For this review, take the finished solid that the model builds, in its own axes (mm). A direction names the side the tool comes from. Round coordinates to 2 decimals unless told otherwise and drop trailing zeros. Write each loop counter-clockwise with the first axis right and the second up, starting at its lowest first coordinate (ties: lowest second). Pieces come first, ordered by that corner, then holes. Notation, with made-up numbers: M 72,-37.75 L 77,-37.75 A21 cw 77,-4.75 Z; hole C 68.5,-32 d2. An arc over 180 degrees is marked long. Use one line per item in the form item = value. Start each with the question number.
Item 1: Add section B-B (x = -88.5). State the section outline as (y, z) points, and give its area (3 significant figures).
Item 2: Add section C-C (y = -21). State the section outline as (x, z) points (1 decimal), and give its area (3 significant figures).
Item 3: For line 1 (Y direction, x = -102, z = -24.5); line 2 (Z direction, x = -55.5, y = -8); line 3 (X direction, y = -12, z = -7.5), list the stretches that pass through material, from the lowest coordinate up. Write a range as [from, to].
Item 4: Add section A-A (z = 3.5). State the section outline as (x, y) points, and give its area (3 significant figures).
Item 5: For P1, Ø3, axis at y = -6.5, z = 33, coming from the -X side; P2, Ø12, axis at y = -48, z = 24, coming from the -X side; P3, Ø2, axis at x = -102, y = -9, coming from the +Z side; P4, Ø4, axis at x = -31, y = -16, coming from the +Z side, all flat-tipped, find the tip position at first contact; note any pin that passes through.
Item 6: For faces 5 (the cylindrical face through (-59.555, -37.744, -48.236)), 6 (the cylindrical face through (-68.197, -6.261, -30.855)), list the 3-axis set-ups (+Z, -Z, +X, -X, +Y, -Y) from which the entire face can be reached by the end or side of a thin tool; tool diameter is ignored.
Item 7: Draft analysis for pull direction X (two halves, no side actions). For faces 1 (the cylindrical face through (-100.82, -37.74, 23.23)), 2 (the cylindrical face through (-18.292, -37.744, 23.233)), 3 (the cylindrical face through (-101.66, -6.26, -30.8)), 4 (the flat face through (-39, 0, 23)), state which applies: released by +X, released by -X, zero draft, split by the parting line, or undercut.
Item 8: Add section D-D (y = -7). State the section outline as (x, z) points, and give its area (3 significant figures).
from build123d import *

# Parameters (mm, degrees)
F0_R     = 50.842383
F0_R_2   = 1.905
F0_R_3   = 31.75
F1_DEPTH = 12.7
F2_DEPTH = 63.5


with BuildPart() as f1:
    # F0 (on Front) → F1 (new body)
    with BuildSketch(Plane.XZ):
        with Locations((-61.314686, 0.139674)):
            Circle(F0_R)
        with Locations((-61.314686, -47.506517)):
            Circle(F0_R_2, mode=Mode.SUBTRACT)
        with Locations((-61.314686, 0.139674)):
            Circle(F0_R_3, mode=Mode.SUBTRACT)
        with Locations((-102.577499, 23.96277)):
            Circle(F0_R_2, mode=Mode.SUBTRACT)
        with Locations((-20.051874, 23.96277)):
            Circle(F0_R_2, mode=Mode.SUBTRACT)
    extrude(amount=F1_DEPTH)

    # F0 (on Front) → F2 (join)
    with BuildSketch(Plane.XZ):
        with Locations((-102.577499, 23.96277)):
            Circle(F0_R_2)
        with Locations((-20.051874, 23.96277)):
            Circle(F0_R_2)
        with Locations((-61.314686, -47.506517)):
            Circle(F0_R_2)
    extrude(amount=F2_DEPTH)


solid = f1.part
Calculated:
q1.outline = M -12.7,-42.82 L 0,-42.82 L 0,-16.26 L -12.7,-16.26 Z; M -12.7,16.54 L 0,16.54 L 0,43.1 L -12.7,43.1 Z
q1.area = 675 mm^2
q2.outline = C -102.6,24 d3.8; C -61.3,-47.5 d3.8; C -20.1,24 d3.8
q2.area = 34.2 mm^2
q3.line_1 = [-12.7, 0]
q3.line_2 = [-50.37, -31.07], [31.35, 50.65]
q3.line_3 = [-111.58, -92.13], [-30.5, -11.05]
q4.outline = M -112.05,-12.7 L -92.89,-12.7 L -92.89,0 L -112.05,0 Z; M -29.74,-12.7 L -10.58,-12.7 L -10.58,0 L -29.74,0 Z
q4.area = 487 mm^2
q5.P1 = -101.33
q5.P2 = -104.48
q5.P3 = 31.92
q5.P4 = through
q6.face_5 = -Y
q6.face_6 = +Y, -Y
q7.face_1 = undercut
q7.face_2 = undercut
q7.face_3 = split by the parting line
q7.face_4 = zero draft
q8.outline = C -61.31,0.14 d101.68; hole C -61.31,0.14 d63.5
q8.area = 4,950 mm^2
